```python
from build123d import *

# Parameters (mm, degrees)
F0_W     = 485.775
F0_H     = 19.05
F0_R     = 1.5875
F0_H_2   = 127
F1_DEPTH = 9.525
F0_H_3   = 9.525
F2_DEPTH = 9.525
F4_R     = 1.5875
F5_DEPTH = 9.525
F3_R     = 1.5875
F6_DEPTH = 9.525


with BuildPart() as f1:
    # F0 (on Right) → F1 (new body)
    with BuildSketch(Plane.YZ):
        with Locations((0, -148.74875)):
            Rectangle(F0_W, F0_H)
        with Locations((-230.1875, -148.74875)):
            Circle(F0_R, mode=Mode.SUBTRACT)
        with Locations((-88.9, -148.74875)):
            Circle(F0_R, mode=Mode.SUBTRACT)
        with Locations((86.36, -148.74875)):
            Circle(F0_R, mode=Mode.SUBTRACT)
        with Locations((230.1875, -148.74875)):
            Circle(F0_R, mode=Mode.SUBTRACT)
        with Locations((0, -75.72375)):
            Rectangle(F0_W, F0_H_2)
        with BuildLine():
            Line((-50.8, -101.12375), (50.8, -101.12375))
            ThreePointArc((50.8, -101.12375), (57.15, -107.47375), (50.8, -113.82375))
            Line((50.8, -113.82375), (-50.8, -113.82375))
            ThreePointArc((-50.8, -113.82375), (-57.15, -107.47375), (-50.8, -101.12375))
        make_face(mode=Mode.SUBTRACT)
    extrude(amount=F1_DEPTH)

    # F0 (on Right) → F2 (join)
    with BuildSketch(Plane.YZ):
        with Locations((0, -75.72375)):
            Rectangle(F0_W, F0_H_2)
        with BuildLine():
            Line((-50.8, -101.12375), (50.8, -101.12375))
            ThreePointArc((50.8, -101.12375), (57.15, -107.47375), (50.8, -113.82375))
            Line((50.8, -113.82375), (-50.8, -113.82375))
            ThreePointArc((-50.8, -113.82375), (-57.15, -107.47375), (-50.8, -101.12375))
        make_face(mode=Mode.SUBTRACT)
        with Locations((0, -7.46125)):
            Rectangle(F0_W, F0_H_3)
    extrude(amount=-F2_DEPTH)

    # F4 (on face) → F5 (cut)
    with BuildSketch(Plane(origin=(0, 242.8875, 0), x_dir=(-1, 0, 0), z_dir=(0, 1, 0))):
        with Locations((0, -43.97375)):
            Circle(F4_R)
        with Locations((0, -113.82375)):
            Circle(F4_R)
    extrude(amount=-F5_DEPTH, mode=Mode.SUBTRACT)

    # F3 (on face) → F6 (cut)
    with BuildSketch(Plane.XZ.offset(242.8875)):
        with Locations((0, -113.82375)):
            Circle(F3_R)
        with Locations((0, -43.97375)):
            Circle(F3_R)
    extrude(amount=-F6_DEPTH, mode=Mode.SUBTRACT)


solid = f1.part
```
Work out the finished part from the listing and answer in its coordinate system (mm). A direction names the side the tool comes from. Give positions to 0.01 mm unless a question says otherwise; leave off trailing zeros. Loops run counter-clockwise (first coordinate to the right, second up) from the corner with the lowest first, then second, coordinate; pieces in that order, holes last. Notation, with made-up numbers: M 33,8.5 L 40,8.5 A21 cw 40,20.5 Z; hole C 29.5,-8 d3. An arc over 180 degrees is marked long. One line per item, written item: value. Start each with the question number.
1. Determine the mould class of faces 1 (the face through (9.525, -3, -84)), 2 (the face through (0, 1, -113.824)), 3 (the face through (0, -242.888, -79)), 4 (the face through (0, 242.888, -82)) for opening direction Y: released by +Y, released by -Y, zero draft, split by the parting line, or undercut.
2. Which of the six approach directions +Z, -Z, +X, -X, +Y, -Y give full straight-line access (tool end or side, diameter ignored) to faces 5 (the face through (0.13, -57.15, -107.61)), 6 (the face through (5, -3, -12.224)), 7 (the face through (5, -3, -158.274)), 8 (the face through (-5, -3, -139.224)), 9 (the face through (-5, -3, -2.699))?
3. Find the intervals of material crossed by probe 1 along Z at (x, y) = (-1.5, 26); probe 2 along Z at (x, y) = (0.5, -49.5); probe 3 along Z at (x, y) = (-1.5, -171.5), in increasing order.
4. Find section A-A (y = 39.5). Give the vertices of the cut face in (x, z) (3 decimals).
5. Find section C-C (y = -66.5). Give the vertices of the cut face in (x, z) (3 decimals), and give its area (3 significant figures).
6. Each of these flat-tipped pins is pushed along its axis until it touches: P1, Ø1.9, axis at x = 0, z = -43.97, coming from the -Y side; P2, Ø3, axis at x = -5, y = -21.5, coming from the -Z side; P3, Ø5, axis at y = -88.9, z = -148.75, coming from the -X side; P4, Ø10.5, axis at y = 54, z = -9, coming from the +X side (3 decimals). Where does it stop, or does it pass through?
7. Find section B-B (x = -4.5). Give the vertices of the cut face in (y, z), and give its area (3 significant figures).
Reported:
1. face 1: zero draft
1. face 2: undercut
1. face 3: released by -Y
1. face 4: released by +Y
2. face 5: +X, -X
2. face 6: +Z, +X, +Y, -Y
2. face 7: -Z, +X, -X, +Y, -Y
2. face 8: -Z, -X, +Y, -Y
2. face 9: +Z, +X, -X, +Y, -Y
3. probe 1: z = -139.22 to -113.82, -101.12 to -2.7
3. probe 2: z = -158.27 to -113.82, -101.12 to -12.22
3. probe 3: z = -139.22 to -2.7
4. outline: M -9.525,-139.224 L 0,-139.224 L 0,-158.274 L 9.525,-158.274 L 9.525,-113.824 L -9.525,-113.824 Z; M -9.525,-101.124 L 9.525,-101.124 L 9.525,-12.224 L 0,-12.224 L 0,-2.699 L -9.525,-2.699 Z
5. outline: M -9.525,-139.224 L 0,-139.224 L 0,-158.274 L 9.525,-158.274 L 9.525,-12.224 L 0,-12.224 L 0,-2.699 L -9.525,-2.699 Z
5. area: 2,690 mm²
6. P1: stops at y = -233.36
6. P2: stops at z = -139.22
6. P3: stops at x = 0
6. P4: stops at x = 9.525
7. outline: M -242.89,-139.22 L 242.89,-139.22 L 242.89,-2.7 L -242.89,-2.7 Z; hole M -50.8,-113.82 L 50.8,-113.82 A6.35 ccw 50.8,-101.12 L -50.8,-101.12 A6.35 ccw Z
7. area: 64,900 mm²
